Here's how the part is built. I have some questions about the finished solid (model axes, mm). Face numbers are marked on the shaded views. A direction names the side the tool comes from. Give positions to 0.01 mm unless a question says otherwise; leave off trailing zeros. Order: outer loops, then holes, each group sorted by start corner. A loop starts at its lowest first (then second) coordinate and runs counter-clockwise, first axis right, second up. Notation, with made-up numbers: (77.5, 19.5) -> (121.5, 19.5) arc R27 ccw to (121.5, 35.5) -> close; hole circle Ø10 at (51, 14.25). An arc over 180 degrees is marked (long way). Write each question's results on one line, items separated by ' | '. Start each with the question number.
Q1. Imagine slicing it at C-C, the plane y = 2. Please give me the cut outline in (x, z).
Q2. I need wall thicknesses on line 1 along Y through (x, z) = (-19.05, 0) (3 decimals); line 2 along Y through (x, z) = (-5.5, 1.75); line 3 along X through (y, z) = (-21, -2.5). Which ranges of each line are inside material? Lowest first, please. Write a range as [from, to].
Q3. Thinking about a two-plate mould opening in Y: for the marked faces 3, 4 and 5, which applies, pulls with the +Y half, pulls with the -Y half, needs draft (parallel to the pull), parting line crosses it, or undercut?
Q4. I'm going to push flat-ended pins straight in: pin 1 (3 mm diameter, centred on x = -52.5, z = -3, fed in from +Y); pin 2 (10 mm diameter, centred on x = -59.5, y = -31, fed in from -Z) (3 decimals); pin 3 (4 mm diameter, centred on x = -16.5, z = -1.5, fed in from +Y); pin 4 (4 mm diameter, centred on x = -44.45, y = -25.4, fed in from +Z) (3 decimals). Where does each tip first touch, or does it pass through?
Q5. Imagine slicing it at D-D, the plane y = -33. Please give me the cut outline in (x, z) (3 decimals), then the cut area to 3 significant figures.
Q6. Imagine slicing it at B-B, the plane z = 0. State how many separate pieces and enclosed holes the cut face has, then the cut area to 3 significant figures.
Q7. For the marked faces 1 and 2, which set-ups out of +Z, -Z, +X, -X, +Y, -Y let a thin tool reach every point of the face, with its end or its side?
```python
from build123d import *

# Parameters (mm, degrees)
BOSS_EXTRUDE1_DEPTH                             = 6.35
SKETCH4_R                                       = 12.7
CUT_EXTRUDE3_DEPTH                              = 116.178567885
SKETCH5_R                                       = 15.875
CUT_EXTRUDE4_DEPTH                              = 4.5085
FILLET1_R                                       = 25.4
F_8_32_TAPPED_HOLE2_D                           = 3.4544
F_8_32_TAPPED_HOLE2_DEPTH                       = 10.668
F_8_32_TAPPED_HOLE2_TIP                         = 1.037806461
F_1_4_20_TAPPED_HOLE1_D                         = 5.1054
SKETCH27_R                                      = 7.9375
CUT_EXTRUDE6_DEPTH                              = 4.572
CUT_EXTRUDE8_START                              = -9.525
CUT_EXTRUDE8_DEPTH                              = 9.525
FILLET2_R                                       = 6.35
F_8_32_TAPPED_HOLE1_D                           = 3.4544
F_8_32_TAPPED_HOLE1_DEPTH                       = 10.668
F_8_32_TAPPED_HOLE1_TIP                         = 1.037806461
F_4_40_TAPPED_HOLE1_D                           = 2.2606
F_4_40_TAPPED_HOLE1_DEPTH                       = 7.62
F_4_40_TAPPED_HOLE1_TIP                         = 0.679152758
CSK_FOR_10_FLAT_HEAD_MACHINE_SCREW1_D           = 5.1054
CSK_FOR_10_FLAT_HEAD_MACHINE_SCREW1_CSINK_D     = 9.779
CSK_FOR_10_FLAT_HEAD_MACHINE_SCREW1_CSINK_ANGLE = 82


with BuildPart() as part:
    # Sketch1 → Boss-Extrude1 (new, symmetric)
    with BuildSketch(Plane.XY):
        with BuildLine():
            Line((25.4, 0), (25.4, -63.5))
            Line((25.4, -63.5), (-95.25, -63.5))
            Line((-95.25, -63.5), (-95.25, -31.75))
            Line((-95.25, -31.75), (-13.866905739, 21.280717216))
            ThreePointArc((-13.866905739, 21.280717216), (12.10249136, 22.33136142), (25.4, 0))
        make_face()
    extrude(amount=BOSS_EXTRUDE1_DEPTH, both=True)

    # Sketch4 → Cut-Extrude3 (cut, through all)
    with BuildSketch(Plane.XY.offset(6.35)):
        Circle(SKETCH4_R)
    extrude(amount=-CUT_EXTRUDE3_DEPTH, mode=Mode.SUBTRACT)

    # Sketch5 → Cut-Extrude4 (cut)
    with BuildSketch(Plane(origin=(0, 0, -6.35), x_dir=(-1, 0, 0), z_dir=(0, 0, -1))):
        Circle(SKETCH5_R)
    extrude(amount=-CUT_EXTRUDE4_DEPTH, mode=Mode.SUBTRACT)

    # Fillet1
    fillet1_edges = [part.edges().sort_by_distance(p)[0] for p in [
        (-95.25, -31.75, 0),
    ]]
    fillet(fillet1_edges, radius=FILLET1_R)

    # #8-32 Tapped Hole2
    with Locations(Plane(origin=(25.4, 0, 0), x_dir=(0, 0, -1), z_dir=(1, 0, 0))):
        with Locations((0, -50.8)):
            Hole(F_8_32_TAPPED_HOLE2_D / 2, depth=F_8_32_TAPPED_HOLE2_DEPTH)
            with Locations((0, 0, -(F_8_32_TAPPED_HOLE2_DEPTH + F_8_32_TAPPED_HOLE2_TIP / 2))):  # 118° drill point
                Cone(0, F_8_32_TAPPED_HOLE2_D / 2, F_8_32_TAPPED_HOLE2_TIP, mode=Mode.SUBTRACT)

    # 1/4-20 Tapped Hole1 (through all)
    with Locations(Plane.XY.offset(6.35)):
        with Locations((-19.05, -19.05)):
            Hole(F_1_4_20_TAPPED_HOLE1_D / 2)

    # Sketch27 → Cut-Extrude6 (cut)
    with BuildSketch(Plane.XY.offset(6.35)):
        with Locations((-19.05, -19.05)):
            Circle(SKETCH27_R)
    extrude(amount=-CUT_EXTRUDE6_DEPTH, mode=Mode.SUBTRACT)

    # Sketch28 → Cut-Extrude8 (cut)
    with BuildSketch(Plane(origin=(0, 0, -6.35), x_dir=(-1, 0, 0), z_dir=(0, 0, -1)).offset(CUT_EXTRUDE8_START)):
        with BuildLine():
            ThreePointArc((5.38883143, -24.821774631), (-7.920985408, -24.133337734), (-19.05, -16.800520825))
            Line((-19.05, -16.800520825), (-19.05, -57.15))
            Line((-19.05, -57.15), (88.9, -57.15))
            Line((88.9, -57.15), (88.9, -45.515541418))
            ThreePointArc((88.9, -45.515541418), (86.598521065, -36.438672898), (80.250179304, -29.555003506))
            Line((80.250179304, -29.555003506), (48.206868735, -8.674994495))
            ThreePointArc((48.206868735, -8.674994495), (35.288934952, -8.113746603), (28.574321085, -19.163722759))
            ThreePointArc((28.574321085, -19.163722759), (23.199392186, -27.623690541), (13.229821608, -26.589970059))
            ThreePointArc((13.229821608, -26.589970059), (9.504977418, -24.838266448), (5.38883143, -24.821774631))
        make_face()
    extrude(amount=CUT_EXTRUDE8_DEPTH, mode=Mode.SUBTRACT)

    # Fillet2
    # the kernel refuses this fillet: 6.35 mm, written as the material it adds along each edge
    with BuildSketch(Plane(origin=(19.05, -57.15, 3.175), x_dir=(0, 1, 0), z_dir=(0, 0, -1))) as fillet2_piece_1_section:
        with BuildLine():
            CenterArc((FILLET2_R, -FILLET2_R), FILLET2_R, 90, 90)
            Line((0, -FILLET2_R), (0, 0))
            Line((0, 0), (FILLET2_R, 0))
        make_face()
    fillet2_piece_1 = extrude(amount=9.525, mode=Mode.PRIVATE)
    fillet2_piece_1 = fillet2_piece_1 - Plane(origin=(17.599243773, -50.8, 0), x_dir=(0, 0, 1), z_dir=(-1, 0, 0)) * Cylinder(1.7272, 45, mode=Mode.PRIVATE)
    add(fillet2_piece_1)
    with BuildSketch(Plane(origin=(-88.9, -57.15, 3.175), x_dir=(1, 0, 0), z_dir=(0, 0, -1))) as fillet2_piece_2:
        with BuildLine():
            CenterArc((FILLET2_R, -FILLET2_R), FILLET2_R, 90, 90)
            Line((0, -FILLET2_R), (0, 0))
            Line((0, 0), (FILLET2_R, 0))
        make_face()
    extrude(amount=9.525)
    with BuildSketch(Plane(origin=(19.05, -16.800520825, 3.175), x_dir=(-0.8081515274529607, -0.5889746248145555, 0), z_dir=(0, 0, -1))) as fillet2_piece_3:
        with BuildLine():
            CenterArc((12.375463834, -6.199333292), FILLET2_R, 102.506099706, 113.578178478)
            Line((7.243701634, -9.93932216), (0, 0))
            ThreePointArc((0, 0), (5.500206148, -0.60266683), (11.000412296, 0))
        make_face()
    extrude(amount=9.525)

    # #8-32 Tapped Hole1
    with Locations(Plane.XZ.offset(63.5)):
        with Locations((12.7, 0), (-34.925, 0), (-82.55, 0)):
            Hole(F_8_32_TAPPED_HOLE1_D / 2, depth=F_8_32_TAPPED_HOLE1_DEPTH)
            with Locations((0, 0, -(F_8_32_TAPPED_HOLE1_DEPTH + F_8_32_TAPPED_HOLE1_TIP / 2))):  # 118° drill point
                Cone(0, F_8_32_TAPPED_HOLE1_D / 2, F_8_32_TAPPED_HOLE1_TIP, mode=Mode.SUBTRACT)

    # #4-40 Tapped Hole1
    with Locations(Plane(origin=(0, 0, 3.175), x_dir=(-1, 0, 0), z_dir=(0, 0, -1))):
        with Locations((-6.35, -43.18)):
            Hole(F_4_40_TAPPED_HOLE1_D / 2, depth=F_4_40_TAPPED_HOLE1_DEPTH)
            with Locations((0, 0, -(F_4_40_TAPPED_HOLE1_DEPTH + F_4_40_TAPPED_HOLE1_TIP / 2))):  # 118° drill point
                Cone(0, F_4_40_TAPPED_HOLE1_D / 2, F_4_40_TAPPED_HOLE1_TIP, mode=Mode.SUBTRACT)

    # CSK for #10 Flat Head Machine Screw1 (through all)
    with Locations(Plane.XY.offset(6.35)):
        with Locations((-44.45, -25.4)):
            CounterSinkHole(CSK_FOR_10_FLAT_HEAD_MACHINE_SCREW1_D / 2, CSK_FOR_10_FLAT_HEAD_MACHINE_SCREW1_CSINK_D / 2, counter_sink_angle=CSK_FOR_10_FLAT_HEAD_MACHINE_SCREW1_CSINK_ANGLE)


solid = part.part
```
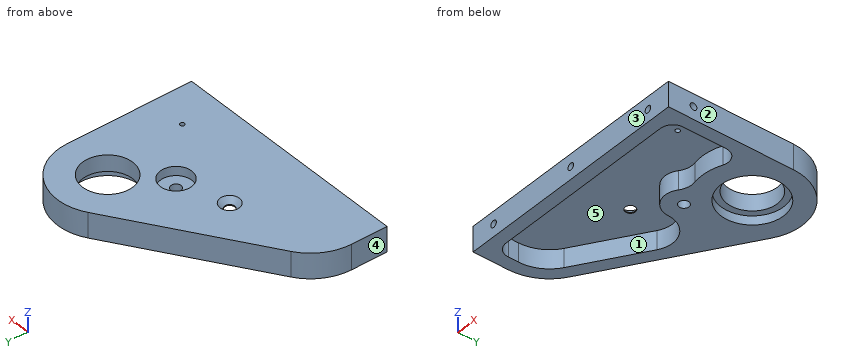
Geometry check:
1) outline: (-43.46, -6.35) -> (-15.75, -6.35) -> (-15.75, -1.84) -> (-12.54, -1.84) -> (-12.54, 6.35) -> (-43.46, 6.35) -> close; (12.54, -1.84) -> (15.75, -1.84) -> (15.75, -6.35) -> (25.32, -6.35) -> (25.32, 6.35) -> (12.54, 6.35) -> close
2) line 1: [-63.5, -57.15], [-28.575, -21.603], [-16.497, 17.903] | line 2: [-63.5, -57.15], [-24.8, -11.45], [11.45, 24.8] | line 3: [-78.75, -67.12], [-28.37, -20.7], [-17.4, 25.4]
3) face 3: pulls with the -Y half | face 4: needs draft | face 5: undercut
4) pin 1: y = -2.92 | pin 2: z = 3.175 | pin 3: y = 20.87 | pin 4: through
5) outline: (-91.953, -6.35) -> (-84.212, -6.35) -> (-84.212, 3.175) -> (19.05, 3.175) -> (19.05, -6.35) -> (25.4, -6.35) -> (25.4, 6.35) -> (-91.953, 6.35) -> close | area: 507 mm²
6) separate pieces: 4 | enclosed holes: 2 | area: 3,570 mm²
7) face 1: -Z | face 2: +Z, -Z, +X, +Y, -Y
